```python
from build123d import *

# Parameters (mm, degrees)
SKETCH1_W            = 18
SKETCH1_H            = 43.5
BOSS_EXTRUDE1_DEPTH  = 2.5
FILLET1_R            = 5
BOSS_EXTRUDE2_DEPTH  = 9.75
SKETCH3_W            = 2
SKETCH3_H            = 14.5
BOSS_EXTRUDE3_DEPTH  = 9.75
M3_CLEARANCE_HOLE1_D = 3.4
SKETCH7_R            = 3.75
CUT_EXTRUDE1_DEPTH   = 26.477931627
FILLET2_R            = 0.05


with BuildPart() as part:
    # Sketch1 → Boss-Extrude1 (new body)
    with BuildSketch(Plane(origin=(0, 0, 0), x_dir=(1, 0, 0), z_dir=(0, 1, 0))):
        Rectangle(SKETCH1_W, SKETCH1_H)
    extrude(amount=BOSS_EXTRUDE1_DEPTH)

    # Fillet1
    fillet1_edges = [part.edges().sort_by_distance(p)[0] for p in [
        (-9, 1.25, -21.75),
        (-9, 1.25, 21.75),
    ]]
    fillet(fillet1_edges, radius=FILLET1_R)

    # Sketch2 → Boss-Extrude2 (add)
    with BuildSketch(Plane.XZ):
        with BuildLine():
            Line((9, -21.75), (-4, -21.75))
            ThreePointArc((-4, -21.75), (-7.535533906, -20.285533906), (-9, -16.75))
            Line((-9, -16.75), (-9, 16.75))
            ThreePointArc((-9, 16.75), (-7.535533906, 20.285533906), (-4, 21.75))
            Line((-4, 21.75), (9, 21.75))
            Line((9, 21.75), (9, 19.75))
            Line((9, 19.75), (-4, 19.75))
            ThreePointArc((-4, 19.75), (-6.121320344, 18.871320344), (-7, 16.75))
            Line((-7, 16.75), (-7, -16.75))
            ThreePointArc((-7, -16.75), (-6.121320344, -18.871320344), (-4, -19.75))
            Line((-4, -19.75), (9, -19.75))
            Line((9, -19.75), (9, -21.75))
        make_face()
    extrude(amount=BOSS_EXTRUDE2_DEPTH)

    # Sketch3 → Boss-Extrude3 (add)
    with BuildSketch(Plane.XZ):
        with Locations((8, 12.5)):
            Rectangle(SKETCH3_W, SKETCH3_H)
        with Locations((8, -12.5)):
            Rectangle(SKETCH3_W, SKETCH3_H)
    extrude(amount=BOSS_EXTRUDE3_DEPTH)

    # M3 Clearance Hole1 (through all)
    with Locations(Plane(origin=(0, 2.5, 0), x_dir=(1, 0, 0), z_dir=(0, 1, 0))):
        with Locations((0, -18.5), (0, 18.5)):
            Hole(M3_CLEARANCE_HOLE1_D / 2)

    # Sketch7 → Cut-Extrude1 (cut, through all)
    with BuildSketch(Plane.XZ):
        with Locations((0, 18.5)):
            Circle(SKETCH7_R)
        with Locations((0, -18.5)):
            Circle(SKETCH7_R)
    extrude(amount=CUT_EXTRUDE1_DEPTH, mode=Mode.SUBTRACT)

    # Fillet2
    fillet2_edges = [part.edges().sort_by_distance(p)[0] for p in [
        (-1.870828693, -4.875, -21.75),
        (1.870828693, -4.875, -21.75),
        (1.870828693, -4.875, 21.75),
        (-1.870828693, -4.875, 21.75),
    ]]
    fillet(fillet2_edges, radius=FILLET2_R)


solid = part.part
```
Input: part model. Units: mm. Frame: model coordinates. A direction names the side the tool comes from. Coordinates: 2 decimals unless noted, no trailing zeros. Write each loop counter-clockwise with the first axis right and the second up, starting at its lowest first coordinate (ties: lowest second). Pieces come first, ordered by that corner, then holes. Notation, with made-up numbers: (59.25, 55.25) - (90.25, 55.25) arc R20 ccw to (90.25, 73.25) - close; hole circle Ø5 at (58, -22). An arc over 180 degrees is marked (long way). Put each result on its own line as item: value. Start each with the question number.
1) Contact query for flat-ended pins moving along their axis: pin 1 (5 mm diameter, centred on x = 4, z = 6, fed in from -Y); pin 2 (1 mm diameter, centred on x = -5.5, y = -1, fed in from -Z); pin 3 (6 mm diameter, centred on x = -6, y = -7, fed in from -Z). Output: stop coordinate, or through.
2) Cut plane D-D (y = -3). Return the cut outline in (x, z), plus the area to 3 significant figures.
3) Cut plane B-B (z = -8). Return the cut outline in (x, y).
4) Cut plane C-C (y = 1.5). Return the cut outline in (x, z), plus the area to 3 significant figures.
5) Mould query, pull axis Z, two halves, no side actions, for faces 1 (the face through (7, -5, -13)), 2 (the face through (4, -4, -21.75)), 3 (the face through (8, -9.75, -15)). Classes: pulls with the +Z half, pulls with the -Z half, needs draft (parallel to the pull), parting line crosses it, or undercut.
6) Ray query, L1, parallel to Z at x = 0, y = 1.15; L2, parallel to Z at x = 7.5, y = -4.5; L3, parallel to Y at x = 2, z = 12. Return the intervals inside material, ascending.
7) Reachability of faces 4 (the face through (8, -5, -5.25)), 5 (the face through (0, 2.5, 0)), 6 (the face through (2.949, -4.807, 20.817)) from +Z, -Z, +X, -X, +Y, -Y: full face, straight path, thin tool, end or side. Return the list, or none.
8) Cut plane A-A (x = 0). Return the cut outline in (y, z).
Resolved:
1. pin 1: stops at y = 0
1. pin 2: stops at z = -21.65
1. pin 3: stops at z = -21.75
2. outline: (-9, -16.75) arc R5 ccw to (-4, -21.75) - (-2.05, -21.75) arc R0.05 ccw to (-2.02, -21.66) arc R3.75 cw to (-3.54, -19.75) - (-4, -19.75) arc R3 cw to (-7, -16.75) - (-7, 16.75) arc R3 cw to (-4, 19.75) - (-3.54, 19.75) arc R3.75 cw to (-2.02, 21.66) arc R0.05 ccw to (-2.05, 21.75) - (-4, 21.75) arc R5 ccw to (-9, 16.75) - close; (2.02, -21.66) arc R0.05 ccw to (2.05, -21.75) - (9, -21.75) - (9, -5.25) - (7, -5.25) - (7, -19.75) - (3.54, -19.75) arc R3.75 cw to start; (2.02, 21.66) arc R3.75 cw to (3.54, 19.75) - (7, 19.75) - (7, 5.25) - (9, 5.25) - (9, 21.75) - (2.05, 21.75) arc R0.05 ccw to start
2. area: 179 mm2
3. outline: (-9, -9.75) - (-7, -9.75) - (-7, 0) - (7, 0) - (7, -9.75) - (9, -9.75) - (9, 2.5) - (-9, 2.5) - close
4. outline: (-9, -16.75) arc R5 ccw to (-4, -21.75) - (9, -21.75) - (9, 21.75) - (-4, 21.75) arc R5 ccw to (-9, 16.75) - close; hole circle Ø3.4 at (0, -18.5); hole circle Ø3.4 at (0, 18.5)
4. area: 754 mm2
5. face 1: undercut
5. face 2: pulls with the -Z half
5. face 3: needs draft
6. L1: z = -21.75 to -20.2, -16.8 to 16.8, 20.2 to 21.75
6. L2: z = -21.75 to -5.25, 5.25 to 21.75
6. L3: y = 0 to 2.5
7. face 4: +X, -Y
7. face 5: +Z, -Z, +X, -X, +Y
7. face 6: -Y
8. outline: (0, -21.75) - (2.5, -21.75) - (2.5, -20.2) - (0, -20.2) - close; (0, -16.8) - (2.5, -16.8) - (2.5, 16.8) - (0, 16.8) - close; (0, 20.2) - (2.5, 20.2) - (2.5, 21.75) - (0, 21.75) - close
